```python
from build123d import *

# Parameters (mm, degrees)
SKETCH2_W           = 29.29
SKETCH2_H           = 29.29
BOSS_EXTRUDE1_DEPTH = 14.645
SKETCH3_R           = 13.825
BOSS_EXTRUDE2_DEPTH = 10.25
SKETCH4_R           = 11.825
CUT_EXTRUDE1_DEPTH  = 10.25


with BuildPart() as part:
    # Sketch2 → Boss-Extrude1 (new body, symmetric)
    with BuildSketch(Plane(origin=(0, 0, 0), x_dir=(1, 0, 0), z_dir=(0, 1, 0))):
        Rectangle(SKETCH2_W, SKETCH2_H)
    extrude(amount=BOSS_EXTRUDE1_DEPTH, both=True)

    # Sketch3 → Boss-Extrude2 (add)
    with BuildSketch(Plane.XY.offset(14.645)):
        Circle(SKETCH3_R)
    extrude(amount=BOSS_EXTRUDE2_DEPTH)

    # Sketch4 → Cut-Extrude1 (cut)
    with BuildSketch(Plane.XY.offset(24.895)):
        Circle(SKETCH4_R)
    extrude(amount=-CUT_EXTRUDE1_DEPTH, mode=Mode.SUBTRACT)


solid = part.part
```
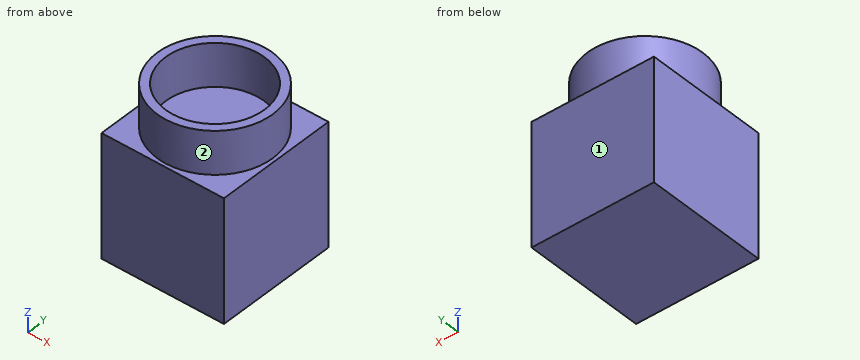
Input: part model. Units: mm. Frame: model coordinates. Face numbers are marked on the shaded views. A direction names the side the tool comes from. Round coordinates to 2 decimals unless told otherwise and drop trailing zeros. Loops run counter-clockwise (first coordinate to the right, second up) from the corner with the lowest first, then second, coordinate; pieces in that order, holes last.
1) Section query C-C on y = 12.5. Return the cut outline in (x, z) (3 decimals).
Ans:
outline: (-14.645, -14.645) - (14.645, -14.645) - (14.645, 14.645) - (5.906, 14.645) - (5.906, 24.895) - (-5.906, 24.895) - (-5.906, 14.645) - (-14.645, 14.645) - close
2) Material intervals for line 1 (Y direction, x = 0, z = 20.5) (3 decimals); line 2 (Z direction, x = -13, y = 9.75) (3 decimals); line 3 (Y direction, x = 12, z = 16.5), sorted ascending.
Ans:
line 1: y = -13.825 to -11.825, 11.825 to 13.825
line 2: z = -14.645 to 14.645
line 3: y = -6.87 to 6.87
3) Section query B-B on x = 9.5. Return the cut outline in (y, z) (3 decimals), plus the area to 3 significant figures.
Ans:
outline: (-14.645, -14.645) - (14.645, -14.645) - (14.645, 14.645) - (10.044, 14.645) - (10.044, 24.895) - (7.041, 24.895) - (7.041, 14.645) - (-7.041, 14.645) - (-7.041, 24.895) - (-10.044, 24.895) - (-10.044, 14.645) - (-14.645, 14.645) - close
area: 919 mm2
4) Section query A-A on y = 0. Return the cut outline in (x, z) (3 decimals), plus the area to 3 significant figures.
Ans:
outline: (-14.645, -14.645) - (14.645, -14.645) - (14.645, 14.645) - (13.825, 14.645) - (13.825, 24.895) - (11.825, 24.895) - (11.825, 14.645) - (-11.825, 14.645) - (-11.825, 24.895) - (-13.825, 24.895) - (-13.825, 14.645) - (-14.645, 14.645) - close
area: 899 mm2
5) Set-up query: the marked faces 1 and 2. Return all of +Z, -Z, +X, -X, +Y, -Y with unobstructed straight access to the full face (end or side cutting, diameter ignored); none if empty.
Ans:
face 1: +Z, -Z, +X, -X, +Y
face 2: +Z
6) Pin query (flat end, axial travel): pin 1 (12 mm diameter, centred on x = 0.5, y = -2, fed in from +Z) (3 decimals). Return the tip coordinate at first contact, or that it passes through.
Ans:
pin 1: stops at z = 14.645
